Verification items for the finished model (mm, model axes). Coordinates: 2 decimals unless noted, no trailing zeros. Order: outer loops, then holes, each group sorted by start corner. A loop starts at its lowest first (then second) coordinate and runs counter-clockwise, first axis right, second up. Notation, with made-up numbers: (-30.75, 70.5) - (16.25, 70.5) arc R15 ccw to (16.25, 92.5) - close; hole circle Ø6 at (-11, 34.25). An arc over 180 degrees is marked (long way). One line per question, with ' | ' between items. Start each with the question number.
from build123d import *

# Parameters (mm, degrees)
SKETCH1_R               = 435
SKETCH1_R_2             = 385
BOSS_EXTRUDE1_DEPTH     = 1.5
CUT_EXTRUDE1_DEPTH      = 616.190214487
CUT_EXTRUDE1_DEPTH_BACK = 616.190214487
SKETCH2_R               = 8


with BuildPart() as part:
    # Sketch1 → Boss-Extrude1 (new, symmetric)
    with BuildSketch(Plane(origin=(0, 0, 0), x_dir=(1, 0, 0), z_dir=(0, 1, 0))):
        with Locations(Location((0, 0, 0), (0, 0, 270))):
            Circle(SKETCH1_R)
        with Locations(Location((0, 0, 0), (0, 0, 270))):
            Circle(SKETCH1_R_2, mode=Mode.SUBTRACT)
    extrude(amount=BOSS_EXTRUDE1_DEPTH, both=True)

    # Sketch2 → Cut-Extrude1 (cut, two sides: drawn at the far end of the back side and taken through both)
    with BuildSketch(Plane(origin=(0, 1.5, 0), x_dir=(1, 0, 0), z_dir=(0, 1, 0)).offset(-CUT_EXTRUDE1_DEPTH_BACK)):
        with Locations(Location((410, 0, 0), (0, 0, 270))):
            Circle(SKETCH2_R)
        with Locations(Location((289.913780286, -289.913780286, 0), (0, 0, 270))):
            Circle(SKETCH2_R)
        with Locations(Location((0, -410, 0), (0, 0, 270))):
            Circle(SKETCH2_R)
        with Locations(Location((-289.913780286, -289.913780286, 0), (0, 0, 270))):
            Circle(SKETCH2_R)
        with Locations(Location((-410, 0, 0), (0, 0, 270))):
            Circle(SKETCH2_R)
        with Locations(Location((-289.913780286, 289.913780286, 0), (0, 0, 270))):
            Circle(SKETCH2_R)
        with Locations(Location((0, 410, 0), (0, 0, 270))):
            Circle(SKETCH2_R)
        with Locations(Location((289.913780286, 289.913780286, 0), (0, 0, 270))):
            Circle(SKETCH2_R)
    extrude(amount=CUT_EXTRUDE1_DEPTH + CUT_EXTRUDE1_DEPTH_BACK, mode=Mode.SUBTRACT)


solid = part.part
Item 1: Section check A-A (z = -140). Record the cut outline in (x, y), then the cut area to 3 significant figures.
Item 2: Section check C-C (y = -1). Give the number of separate pieces and of enclosed holes in the cut face, then the cut area to 3 significant figures.
Item 3: Thickness scan on probe 1 along X at (y, z) = (-0.7, 0); probe 2 along X at (y, z) = (-0.55, 285); probe 3 along Z at (x, y) = (184, -0.05). Record the ranges inside material, lowest first. Write a range as from..to.
Item 4: Section check B-B (x = 322.5). Record the cut outline in (y, z).
Item 5: Mould release check, pull along Z, two halves, no side actions. Record for faces 1 (the flat face through (-385, -1.5, 30)), 2 (the cylindrical face through (-424.656, 0.021, -94.299)), 3 (the cylindrical face through (-234.27, -0.02, -305.52)): +Z half, -Z half, draft (parallel to the pull), parting line (faces both ways), or undercut.
Completed:
1) outline: (-411.86, -1.5) - (-358.64, -1.5) - (-358.64, 1.5) - (-411.86, 1.5) - close; (358.64, -1.5) - (411.86, -1.5) - (411.86, 1.5) - (358.64, 1.5) - close | area: 319 mm^2
2) separate pieces: 1 | enclosed holes: 9 | area: 127,000 mm^2
3) probe 1: x = -435..-418, -402..-385, 385..402, 418..435 | probe 2: x = -328.63..-296.23, -283.6..-258.84, 258.84..283.6, 296.23..328.63 | probe 3: z = -394.17..-338.18, 338.18..394.17
4) outline: (-1.5, -291.92) - (1.5, -291.92) - (1.5, -210.28) - (-1.5, -210.28) - close; (-1.5, 210.28) - (1.5, 210.28) - (1.5, 291.92) - (-1.5, 291.92) - close
5) face 1: draft | face 2: parting line | face 3: undercut
